Design review of the part built by this model. Coordinates are the model's own, in mm. A direction names the side the tool comes from. Coordinates: 2 decimals unless noted, no trailing zeros. Write each loop counter-clockwise with the first axis right and the second up, starting at its lowest first coordinate (ties: lowest second). Pieces come first, ordered by that corner, then holes.
Q1. Add section D-D, the plane z = 18. Give the boundary of the cut face in (x, y).
Q2. Clearance check with flat-ended pins moving along their axes: pin 1 Ø3.5 at (x, y) = (-492.41, 207.52) entering from +Z; pin 2 Ø1 at (x, z) = (-500.5, 4) entering from -Y; pin 3 Ø2.5 at (x, y) = (-401.06, 232.12) entering from -Z; pin 4 Ø2 at (y, z) = (231.5, 1) entering from -X. State where each tip first meets the part, or that it passes through.
Q3. Add section C-C, the plane x = -456.5. Give the boundary of the cut face in (y, z).
Q4. The part is to be moulded in two halves that separate along Z. For faces 6 (the face through (-500.72, 209.31, 6.29)), 7 (the face through (-496.059, 217, 21)), 8 (the face through (-500.496, 217.618, 20.643)), say which applies: +Z half, -Z half, draft (parallel to the pull), parting line (faces both ways), or undercut.
Q5. Add section B-B, the plane z = 13.75. Give the boundary of the cut face in (x, y), plus the area to 3 significant figures.
Q6. To check wall thickness, follow probe 1 along Y at (x, z) = (-500.75, 12.4); probe 2 along X at (y, z) = (233, 1.5); probe 3 along Z at (x, y) = (-450, 199.5). State the ranges of each line that lie inside material, in increasing order.
Q7. Machinability: for faces 1 (the face through (-496.259, 209, 3)), 2 (the face through (-500.72, 209.36, 18.69)), 3 (the face through (-500, 217, 2.958)), 4 (the face through (-496.259, 226, 5)), 5 (the face through (-496.059, 233, 1)), which of the approach directions +Z, -Z, +X, -X, +Y, -Y give a long, thin tool a straight path to every point of the face, cutting with its end or side? Answer none if there is none.
Q8. Add section A-A, the plane y = 220. Give the boundary of the cut face in (x, z).
from build123d import *

# Parameters (mm, degrees)
SKETCH1_W               = 100
SKETCH1_H               = 45
SKETCH1_R               = 1.5
BOSS_EXTRUDE2_DEPTH     = 2.5
CUT_EXTRUDE2_DEPTH      = 13
CUT_EXTRUDE2_DEPTH_BACK = 17
SKETCH2_R               = 1.5
SKETCH3_W               = 9
SKETCH3_H               = 19.5
BOSS_EXTRUDE3_DEPTH     = 24.8
CUT_EXTRUDE3_DEPTH      = 8.8
SKETCH7_R               = 8.25
CUT_EXTRUDE4_DEPTH      = 714.8
SKETCH8_W               = 1.252352654
SKETCH8_H               = 2
CUT_EXTRUDE5_DEPTH      = 714.8


with BuildPart() as part:
    # Sketch1 → Boss-Extrude2 (new body)
    with BuildSketch(Plane.XY):
        with Locations((-446.059405941, 217.618811881)):
            Rectangle(SKETCH1_W, SKETCH1_H)
        with Locations((-491.059405941, 232.118811881)):
            Circle(SKETCH1_R, mode=Mode.SUBTRACT)
        with Locations((-491.059405941, 203.118811881)):
            Circle(SKETCH1_R, mode=Mode.SUBTRACT)
        with Locations(Location((-401.059405941, 203.118811881, 0), (0, 0, 180))):
            Circle(SKETCH1_R, mode=Mode.SUBTRACT)
        with Locations(Location((-401.059405941, 232.118811881, 0), (0, 0, 180))):
            Circle(SKETCH1_R, mode=Mode.SUBTRACT)
    extrude(amount=BOSS_EXTRUDE2_DEPTH)

    # Sketch2 → Cut-Extrude2 (cut, two sides: drawn at the far end of the back side and taken through both)
    with BuildSketch(Plane.XY.offset(2.5).offset(-CUT_EXTRUDE2_DEPTH_BACK)):
        with Locations((-436.059405941, 211.918811881)):
            Circle(SKETCH2_R)
        with Locations((-401.059405941, 227.018811881)):
            Circle(SKETCH2_R)
        with Locations((-401.059405941, 207.518811881)):
            Circle(SKETCH2_R)
        with Locations((-492.409405941, 207.518811881)):
            Circle(SKETCH2_R)
        with Locations((-492.409405941, 227.018811881)):
            Circle(SKETCH2_R)
    extrude(amount=CUT_EXTRUDE2_DEPTH + CUT_EXTRUDE2_DEPTH_BACK, mode=Mode.SUBTRACT)

    # Sketch3 → Boss-Extrude3 (add)
    with BuildSketch(Plane.XY):
        with Locations((-500.559405941, 217.268811881)):
            Rectangle(SKETCH3_W, SKETCH3_H)
    extrude(amount=BOSS_EXTRUDE3_DEPTH)

    # Sketch4 → Cut-Extrude3 (cut)
    with BuildSketch(Plane.ZY.offset(505.059405941)):
        Polygon((0, 225.268811881), (0, 223.569543899), (12.4, 227.018811881), (0, 227.018811881), align=None)
        Polygon((24.8, 227.018811881), (12.4, 227.018811881), (24.8, 223.569543899), align=None)
        Polygon((24.8, 211.150624905), (12.4, 207.518811881), (24.8, 207.518811881), align=None)
        Polygon((12.4, 207.518811881), (0, 211.150624905), (0, 209.268811881), (0, 207.518811881), align=None)
    extrude(amount=-CUT_EXTRUDE3_DEPTH, mode=Mode.SUBTRACT)

    # Sketch7 → Cut-Extrude4 (cut)
    with BuildSketch(Plane(origin=(0, 0, 0), x_dir=(0, 0, -1), z_dir=(1, 0, 0))):
        with Locations((-12.4, 217.268811881)):
            Circle(SKETCH7_R)
    extrude(amount=-CUT_EXTRUDE4_DEPTH, mode=Mode.SUBTRACT)

    # Sketch8 → Cut-Extrude5 (cut)
    with BuildSketch(Plane(origin=(0, 0, 0), x_dir=(0, 0, -1), z_dir=(1, 0, 0))):
        with Locations((-3.584653996, 217.268811881)):
            Rectangle(SKETCH8_W, SKETCH8_H)
    extrude(amount=-CUT_EXTRUDE5_DEPTH, mode=Mode.SUBTRACT)


solid = part.part
Here are the results:
1. outline: (-505.06, 209.16) - (-496.26, 209.16) - (-496.26, 207.52) - (-496.06, 207.52) - (-496.06, 211.21) - (-505.06, 211.21) - close; (-505.06, 223.33) - (-496.06, 223.33) - (-496.06, 227.02) - (-496.26, 227.02) - (-496.26, 225.46) - (-505.06, 225.46) - close
2. pin 1: stops at z = 2.5
2. pin 2: stops at y = 209.83
2. pin 3: passes through
2. pin 4: stops at x = -496.06
3. outline: (195.12, 0) - (240.12, 0) - (240.12, 2.5) - (195.12, 2.5) - close
4. face 6: -Z half
4. face 7: draft
4. face 8: undercut
5. outline: (-505.06, 207.91) - (-496.26, 207.91) - (-496.26, 207.52) - (-496.06, 207.52) - (-496.06, 209.13) - (-505.06, 209.13) - close; (-505.06, 225.41) - (-496.06, 225.41) - (-496.06, 227.02) - (-496.26, 227.02) - (-496.26, 226.64) - (-505.06, 226.64) - close
5. area: 22.2 mm2
6. probe 1: y = 207.52 to 209.02, 225.52 to 227.02
6. probe 2: x = -496.06 to -492.27, -489.85 to -402.27, -399.85 to -396.06
6. probe 3: z = 0 to 2.5
7. face 1: -Z, -X, -Y
7. face 2: +Z, -X, -Y
7. face 3: +X, -X
7. face 4: -Z, -X, +Y
7. face 5: +Z, -Z, -X, +Y
8. outline: (-505.06, 0) - (-396.06, 0) - (-396.06, 2.5) - (-496.06, 2.5) - (-496.06, 4.62) - (-505.06, 4.62) - close; (-505.06, 20.18) - (-496.06, 20.18) - (-496.06, 24.8) - (-505.06, 24.8) - close
